Design review of the part built by this model. Coordinates are the model's own, in mm. Coordinates: 2 decimals unless noted, no trailing zeros. Order: outer loops, then holes, each group sorted by start corner. A loop starts at its lowest first (then second) coordinate and runs counter-clockwise, first axis right, second up. Notation, with made-up numbers: M -7.5,80.25 L 37.5,80.25 A7 cw 37.5,89.25 Z; hole C -26,47.25 d9. An arc over 180 degrees is marked long. Use CSV: the item, a comma, the result in double quotes.
Autodesk Inventor part; units mm, degrees
ref_plane "YZ Plane" through (0, 0, 0) normal (1, 0, 0) x (0, 1, 0)
ref_plane "XZ Plane" through (0, 0, 0) normal (0, 1, 0) x (-1, 0, 0)
ref_plane "XY Plane" through (0, 0, 0) normal (0, 0, 1) x (1, 0, 0)
sketch "Szkic1" plane through (0, 0, 0) normal (0, 0, 1) x (1, 0, 0)
  line L0 (0, 0) -> (64, 0) construction
  line L1 (64, 0) -> (64, 64) construction
  line L2 (64, 64) -> (0, 64) construction
  line L3 (0, 64) -> (0, 0) construction
  line L4 (0, 0) -> (168, 0) construction
  line L5 (168, 0) -> (168, 168) construction
  line L6 (168, 168) -> (0, 168) construction
  line L7 (0, 168) -> (0, 0) construction
  line L8 (84, 168) -> (84, 0) construction
  circle A0 centre (84, 84) radius 65 construction
  line L9 (0, 0) -> (64, 0)
  line L10 (64, 0) -> (64, 22.1534)
  line L11 (0, 0) -> (0, 64)
  line L12 (0, 64) -> (22.1534, 64)
  arc A1 (22.1534, 64) -> (64, 22.1534) centre (84, 84) ccw
  dimension "d7" = 64
  dimension "d8" = 64
  dimension "d9" = 168
  dimension "d10" = 168
  dimension "d11" = 130
  dimension "d12" = 64
  dimension "d13" = 64
extrude "Wyciągnięcie proste1" add sketch "Szkic1" along normal blind 6
equation "\"d7\" = d8"
properties part number "Naroznik_54x54"
(1) Clearance check with flat-ended pins moving along their axes: P1, Ø2, axis at x = 54, z = 1, coming from the +Y side; P2, Ø12, axis at x = 17.5, y = 43.5, coming from the -Z side. State where each tip first meets the part, or that it passes through.
The answers:
P1,"stops at y = 26.87"
P2,"stops at z = 0"
(2) Add section A-A on z = 3.15. State the section outline as (x, y) points, and give its area (3 significant figures).
The answers:
outline,"M 0,0 L 64,0 L 64,22.15 A65 cw 22.15,64 L 0,64 Z"
area,"2,940 mm2"
(3) Wall thickness on probe 1 along X at (y, z) = (40, 2); probe 2 along Y at (x, z) = (41, 1.7); probe 3 along X at (y, z) = (39, 1.15): over which ranges is each line inside the solid? List them lowest first.
The answers:
probe 1,"x = 0 to 36.16"
probe 2,"y = 0 to 35.26"
probe 3,"x = 0 to 37.1"
(4) Add section B-B on y = 53. State the section outline as (x, z) points, and give its area (3 significant figures).
The answers:
outline,"M 0,0 L 26.87,0 L 26.87,6 L 0,6 Z"
area,"161 mm2"
(5) Add section C-C on x = 39.5. State the section outline as (y, z) points, and give its area (3 significant figures).
The answers:
outline,"M 0,0 L 36.62,0 L 36.62,6 L 0,6 Z"
area,"220 mm2"
